Geometry check sheet. Reference: the model listing, model coordinates, mm. A direction names the side the tool comes from. Give positions to 0.01 mm unless a question says otherwise; leave off trailing zeros. Order: outer loops, then holes, each group sorted by start corner. A loop starts at its lowest first (then second) coordinate and runs counter-clockwise, first axis right, second up. Notation, with made-up numbers: M 88.5,25 L 139.5,25 A28 cw 139.5,46 Z; hole C -18,72.25 d2. An arc over 180 degrees is marked long. Use CSV: the item, a comma, the result in double quotes. Start each with the question number.
Autodesk Fusion 360 part; units mm, degrees
sketch "Sketch1" plane through (0, 0, 0) normal (0, 0, 1) x (1, 0, 0)
  line L0 (-45, 35) -> (45, 35)
  line L1 (45, 35) -> (45, -35)
  line L2 (45, -35) -> (-45, -35)
  line L3 (-45, -35) -> (-45, 35)
  line L4 (-45, 35) -> (45, -35) construction
  line L5 (45, 35) -> (-45, -35) construction
  line L6 (-35, 25) -> (35, 25)
  line L7 (35, 25) -> (35, -25)
  line L8 (35, -25) -> (-35, -25)
  line L9 (-35, -25) -> (-35, 25)
  line L10 (-35, 25) -> (35, -25) construction
  line L11 (35, 25) -> (-35, -25) construction
  dimension "d1" = 90
  dimension "d2" = 70
  dimension "d3" = 10
  dimension "d4" = 10
extrude "Extrude1" add sketch "Sketch1" along normal blind 5
sketch "Sketch2" plane through (0, -35, 0) normal (0, -1, 0) x (1, 0, 0)
  line L0 (-45, 0) -> (45, 0)
  line L1 (45, 0) -> (45, 5)
  line L2 (45, 5) -> (-45, 5)
  line L3 (-33, 0) -> (-30, 4)
  line L4 (-30, 4) -> (-27, 0)
  line L5 (-33, 0) -> (-27, 0)
  dimension "d37" = 4
  dimension "d40" = 15
  dimension "d41" = 6
extrude "Extrude2" cut sketch "Sketch2" against normal through all
pattern_linear "R-Pattern1" count 4 spacing 20 along (1, 0, 0) of "Extrude2"
sketch "Sketch3" plane through (-45, 0, 0) normal (-1, 0, 0) x (0, -1, 0)
  line L0 (-35, 0) -> (35, 0)
  line L1 (35, 0) -> (35, 5)
  line L2 (35, 5) -> (-35, 5)
  line L3 (-23, 0) -> (-20, 4)
  line L4 (-20, 4) -> (-17, 0)
  dimension "d42" = 6
  dimension "d43" = 4
  dimension "d44" = 15
extrude "Extrude3" cut sketch "Sketch3" against normal through all
pattern_linear "R-Pattern2" count 3 spacing 20 along (0, -1, 0) of "Extrude3"
sketch "Sketch4" plane through (0, 0, 5) normal (0, 0, 1) x (-1, 0, 0)
  line L0 (45, -35) -> (45, 35)
  line L1 (45, 35) -> (-45, 35)
  line L2 (-35, 25) -> (35, 25)
  line L3 (35, 25) -> (35, -25)
  circle A0 centre (40, 30) radius 2
  line L4 (35, -25) -> (-35, -25)
  line L5 (-35, -25) -> (-35, 25)
  line L6 (-45, 35) -> (-45, -35)
  line L7 (-45, -35) -> (45, -35)
  dimension "d23" = 5
  dimension "d24" = 5
  dimension "d25" = 4
extrude "Extrude4" add sketch "Sketch4" along normal blind 2 draft -30 contours A0
sketch "Sketch5" plane through (0, 0, 0) normal (0, 0, -1) x (1, 0, 0)
  circle A0 centre (-40, 30) radius 2
  line L0 (45, -23) -> (35, -23)
  line L1 (-45, 35) -> (-45, 23)
  line L2 (33, -35) -> (45, -35)
  line L3 (-33, 25) -> (-33, 35)
  line L4 (35, -25) -> (33, -25)
  line L5 (-35, 23) -> (-35, 25)
  line L6 (35, -23) -> (35, -25)
  line L7 (33, -25) -> (33, -35)
  line L8 (45, -35) -> (45, -23)
  line L9 (-33, 35) -> (-45, 35)
  line L10 (-45, 35) -> (-45, 23)
  line L11 (-45, 23) -> (-35, 23)
  line L12 (-35, 25) -> (-33, 25)
  line L13 (-33, 35) -> (-45, 35)
  line L14 (35, 23) -> (45, 23)
  line L15 (45, 23) -> (45, 35)
  line L16 (45, 35) -> (33, 35)
  line L17 (33, 35) -> (33, 25)
  line L18 (33, 25) -> (35, 25)
  line L19 (35, 25) -> (35, 23)
  line L20 (-35, -23) -> (-45, -23)
  line L21 (-45, -23) -> (-45, -35)
  line L22 (-45, -35) -> (-33, -35)
  line L23 (-33, -35) -> (-33, -25)
  line L24 (-33, -25) -> (-35, -25)
  line L25 (-35, -25) -> (-35, -23)
  dimension "d30" = 4
  dimension "d45" = 5
  dimension "d46" = 5
extrude "Extrude5" cut sketch "Sketch5" against normal blind 2 draft -30 contours A0
pattern_linear "R-Pattern3" count 2 spacing 80 along (1, 0, 0) count 2 spacing 60 along (0, 1, 0) of "Extrude4", "Extrude5"
(1) Thickness scan on line 1 (X direction, y = 0.5, z = 3.5); line 2 (Y direction, x = -32, z = 2.25); line 3 (Y direction, x = 39.5, z = 3). Record the ranges inside material, lowest first.
(2) Sectioned sample at B-B on z = 1. Give the number of separate pieces and of enclosed holes in the cut face, then the cut area to 3 significant figures.
(3) Access from +Z, -Z, +X, -X, +Y, -Y to the whole of each face (thin tool, end or side, straight path). Record for faces 1 (the face through (-40.1, -21.5, 2)), 2 (the face through (0, 25, 2)), 3 (the face through (8.5, 29.9, 2)).
(4) Draft check along X on faces 4 (the face through (0, -25, 2)), 5 (the face through (0, -30, 0)). Enter one of: +X half, -X half, draft (parallel to the pull), parting line (faces both ways), or undercut.
(5) Sectioned sample at A-A on x = 8.5. Record the cut outline in (y, z), then the cut area to 3 significant figures.
(6) Go/stop test with flat-tipped pins: P1, Ø1.9, axis at x = -40, y = 30, coming from the -Z side; P2, Ø0.8, axis at x = 40, y = 30, coming from the -Z side. Record where each tip stops, or that it passes through.
Responses:
1,line 1,"-45 to -35, 35 to 45"
1,line 2,"-35 to -25, 25 to 35"
1,line 3,"-35 to -20.75, -19.25 to -0.75, 0.75 to 19.25, 20.75 to 35"
2,separate pieces,"14"
2,enclosed holes,"4"
2,area,"2,140 mm2"
3,face 1,"-Z, +X, -X"
3,face 2,"+Z, -Z"
3,face 3,"-Z, +Y, -Y"
4,face 4,"undercut"
4,face 5,"draft"
5,outline,"M -35,2 L -25,2 L -25,5 L -35,5 Z; M 25,2 L 35,2 L 35,5 L 25,5 Z"
5,area,"60.0 mm2"
6,P1,"z = 1.82"
6,P2,"z = 2"
